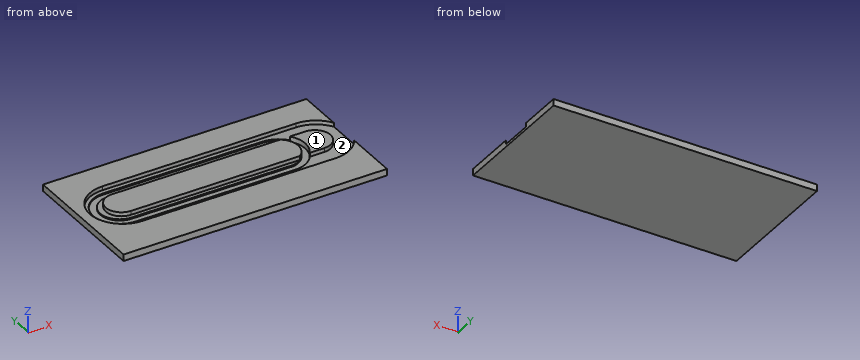
```python
from build123d import *

# Parameters (mm, degrees)
F0_W     = 2000
F0_H     = 1000
F1_DEPTH = 50
F3_DEPTH = 30
F5_DEPTH = 40


with BuildPart() as f1:
    # F0 (on Top) → F1 (new body)
    with BuildSketch(Plane.XY):
        with Locations((29.7885835171, -55.6066778026)):
            Rectangle(F0_W, F0_H)
    extrude(amount=F1_DEPTH)

    # F2 (on face) → F3 (cut)
    with BuildSketch(Plane.XY.offset(50)):
        with BuildLine():
            Line((816.4165019989, 225.2072840929), (-652.1881222725, 225.2072840929))
            ThreePointArc((-652.1881222725, 225.2072840929), (-899.8625352979, -22.4671289325), (-652.1881222725, -270.1415419579))
            Line((-652.1881222725, -270.1415419579), (816.4165019989, -270.1415419579))
            ThreePointArc((816.4165019989, -270.1415419579), (939.2897686207, -237.5131128921), (1029.7885835171, -148.2247119884))
            Line((1029.7885835171, -148.2247119884), (1029.7885835171, 103.2904541234))
            ThreePointArc((1029.7885835171, 103.2904541234), (939.2897686207, 192.5788550272), (816.4165019989, 225.2072840929))
        make_face()
        with BuildLine():
            Line((816.4165019989, -127.1182894707), (-652.1881222725, -127.1182894707))
            ThreePointArc((-652.1881222725, -127.1182894707), (-770.7927748561, -8.5136368871), (-652.1881222725, 110.0910156965))
            Line((-652.1881222725, 110.0910156965), (816.4165019989, 110.0910156965))
            ThreePointArc((816.4165019989, 110.0910156965), (935.0211545825, -8.5136368871), (816.4165019989, -127.1182894707))
        make_face(mode=Mode.SUBTRACT)
    extrude(amount=-F3_DEPTH, mode=Mode.SUBTRACT)

    # F4 (on face) → F5 (cut)
    with BuildSketch(Plane.XY.offset(50)):
        with BuildLine():
            Line((539.0909314156, 190.3235763311), (-666.1416292191, 190.3235763311))
            ThreePointArc((-666.1416292191, 190.3235763311), (-867.5951212645, -11.1299157143), (-666.1416292191, -212.5834077597))
            Line((-666.1416292191, -212.5834077597), (565.2537345886, -212.5834077597))
            ThreePointArc((565.2537345886, -212.5834077597), (740.9686977118, 1.1295941099), (539.0909314156, 190.3235763311))
        make_face()
        with BuildLine():
            Line((561.7653727531, -156.7694544792), (-666.1416292191, -156.7694544792))
            ThreePointArc((-666.1416292191, -156.7694544792), (-813.5253489017, -9.3857347965), (-666.1416292191, 137.9979848862))
            Line((-666.1416292191, 137.9979848862), (540.835082531, 137.9979848862))
            ThreePointArc((540.835082531, 137.9979848862), (688.589879711, 0.362669805), (561.7653727531, -156.7694544792))
        make_face(mode=Mode.SUBTRACT)
    extrude(amount=-F5_DEPTH, mode=Mode.SUBTRACT)


solid = f1.part
```
Could you check a few things on this model? Use its own coordinates, in mm. Face numbers are marked on the shaded views. A direction names the side the tool comes from. Coordinates: 2 decimals unless noted, no trailing zeros. Write each loop counter-clockwise with the first axis right and the second up, starting at its lowest first coordinate (ties: lowest second). Pieces come first, ordered by that corner, then holes. Notation, with made-up numbers: (67.25, 8) -> (114.25, 8) arc R7 cw to (114.25, 21) -> close; hole circle Ø8 at (32, 71). An arc over 180 degrees is marked (long way). One line per question, with ' | ' between items. Start each with the question number.
1. If we section it at B-B (x = -8.5): Please give me the cut outline in (y, z), and give its area (3 significant figures).
2. If we section it at A-A (z = 40.5): Please give me the cut outline in (x, y).
3. Please list where these lines run through material, in increasing order: line 1 along Y through (x, z) = (-286.5, 27.5); line 2 along Y through (x, z) = (-5, 13); line 3 along X through (y, z) = (-8, 13.5).
4. If we section it at D-D (x = 854.5): Please give me the cut outline in (y, z), and give its area (3 significant figures).
5. Will this pin go through, and if not, where does the flat tip stop? P1, Ø10, axis at x = 663, y = -205.5, coming from the +Z side.
6. For the marked faces 1 and 2, which set-ups out of +Z, -Z, +X, -X, +Y, -Y let a thin tool reach every point of the face, with its end or its side?
7. If we section it at C-C (y = -249): Please give me the cut outline in (x, z).
Return value:
1) outline: (-555.61, 0) -> (444.39, 0) -> (444.39, 50) -> (225.21, 50) -> (225.21, 20) -> (190.32, 20) -> (190.32, 10) -> (138, 10) -> (138, 20) -> (110.09, 20) -> (110.09, 50) -> (-127.12, 50) -> (-127.12, 20) -> (-156.77, 20) -> (-156.77, 10) -> (-212.58, 10) -> (-212.58, 20) -> (-270.14, 20) -> (-270.14, 50) -> (-555.61, 50) -> close | area: 41,200 mm²
2) outline: (-970.21, -555.61) -> (1029.79, -555.61) -> (1029.79, -148.22) arc R247.67 cw to (816.42, -270.14) -> (-652.19, -270.14) arc R247.67 cw to (-652.19, 225.21) -> (816.42, 225.21) arc R247.67 cw to (1029.79, 103.29) -> (1029.79, 444.39) -> (-970.21, 444.39) -> close; (-652.19, -127.12) -> (631.69, -127.12) arc R148.13 ccw to (627.37, 110.09) -> (-652.19, 110.09) arc R118.6 ccw to start; (700.41, 110.09) arc R202.3 cw to (705.43, -127.12) -> (816.42, -127.12) arc R118.6 ccw to (816.42, 110.09) -> close
3) line 1: y = -555.61 to -270.14, -127.12 to 110.09, 225.21 to 444.39 | line 2: y = -555.61 to -212.58, -156.77 to 138, 190.32 to 444.39 | line 3: x = -970.21 to -867.57, -813.52 to 688.95, 741.35 to 1029.79
4) outline: (-555.61, 0) -> (444.39, 0) -> (444.39, 50) -> (222.26, 50) -> (222.26, 20) -> (103.81, 20) -> (103.81, 50) -> (-120.84, 50) -> (-120.84, 20) -> (-267.2, 20) -> (-267.2, 50) -> (-555.61, 50) -> close | area: 42,100 mm²
5) P1: stops at z = 20
6) face 1: +Z, +X, -X, +Y, -Y | face 2: +Z
7) outline: (-970.21, 0) -> (1029.79, 0) -> (1029.79, 50) -> (916.54, 50) -> (916.54, 20) -> (-752.32, 20) -> (-752.32, 50) -> (-970.21, 50) -> close
